Work out the finished part from the listing and answer in its coordinate system (mm). Round coordinates to 2 decimals unless told otherwise and drop trailing zeros. Write each loop counter-clockwise with the first axis right and the second up, starting at its lowest first coordinate (ties: lowest second). Pieces come first, ordered by that corner, then holes. Notation, with made-up numbers: (-34.75, 18) -> (-15.75, 18) arc R13 ccw to (-15.75, 40) -> close; hole circle Ø7 at (89, -24.75). An arc over 180 degrees is marked (long way). One line per item, written item: value.
Autodesk Fusion 360 part; units mm, degrees
sketch "スケッチ1" plane through (0, 0, 0) normal (0, 1, 0) x (1, 0, 0)
  line L0 (0, 0) -> (74, 0)
  line L1 (74, 0) -> (74, -44)
  line L2 (74, -44) -> (0, -44)
  line L3 (0, -44) -> (0, 0)
  dimension "d1" = 74
  dimension "d2" = 44
extrude "押し出し1" add sketch "スケッチ1" along normal blind 2
sketch "スケッチ2" plane through (0, 0, 0) normal (0, -1, 0) x (1, 0, 0)
  line L0 (74, 44) -> (0, 44)
  line L1 (0, 44) -> (0, 0)
  line L2 (0, 0) -> (74, 0)
  line L3 (74, 0) -> (74, 44)
  line L4 (72, 37) -> (74, 37)
  line L5 (74, 37) -> (74, 31)
  line L6 (74, 31) -> (72, 31)
  line L7 (72, 31) -> (72, 37)
  line L8 (74, 25) -> (74, 19)
  line L9 (74, 19) -> (72, 19)
  line L10 (72, 19) -> (72, 25)
  line L11 (72, 25) -> (74, 25)
  line L12 (74, 13) -> (74, 7)
  line L13 (74, 7) -> (72, 7)
  line L14 (72, 7) -> (72, 13)
  line L15 (72, 13) -> (74, 13)
  line L16 (2, 25) -> (2, 19)
  line L17 (2, 31) -> (0, 31)
  line L18 (2, 37) -> (2, 31)
  line L19 (0, 25) -> (2, 25)
  line L20 (2, 13) -> (2, 7)
  line L21 (0, 19) -> (0, 25)
  line L22 (0, 13) -> (2, 13)
  line L23 (2, 7) -> (0, 7)
  line L24 (0, 31) -> (0, 37)
  line L25 (0, 37) -> (2, 37)
  line L26 (0, 7) -> (0, 13)
  line L27 (2, 19) -> (0, 19)
  line L28 (74, 44) -> (72, 44)
  line L29 (72, 44) -> (72, 42)
  line L30 (72, 42) -> (74, 42)
  line L31 (74, 42) -> (74, 44)
  line L32 (0, 44) -> (2, 44)
  line L33 (2, 44) -> (2, 42)
  line L34 (2, 42) -> (0, 42)
  line L35 (0, 42) -> (0, 44)
  line L36 (0, 0) -> (2, 0)
  line L37 (2, 0) -> (2, 2)
  line L38 (2, 2) -> (0, 2)
  line L39 (0, 2) -> (0, 0)
  line L40 (74, 0) -> (72, 0)
  line L41 (72, 0) -> (72, 2)
  line L42 (72, 2) -> (74, 2)
  line L43 (74, 2) -> (74, 0)
  dimension "d7" = 0
  dimension "d8" = -12
  dimension "d9" = 2
  dimension "d10" = 7
  dimension "d11" = 6
  dimension "d12" = 6
  dimension "d13" = 7
  dimension "d16" = -72
  dimension "d17" = 0
extrude "押し出し2" cut sketch "スケッチ2" against normal blind 2 contours L0 L3 L28 L29 L30 L31 | L0 L1 L32 L33 L34 L35 | L3 L4 L5 L6 L7 | L3 L8 L9 L10 L11 | L1 L17 L18 L24 L25 | L3 L12 L13 L14 L15 | L1 L16 L19 L21 L27 | L2 L3 L40 L41 L42 L43 | L1 L20 L22 L23 L26 | L1 L2 L36 L37 L38 L39
sketch "スケッチ3" plane through (0, 0, 0) normal (0, -1, 0) x (1, 0, 0)
  line L0 (74, 31) -> (72, 31)
  line L1 (72, 31) -> (72, 37)
  line L2 (72, 37) -> (74, 37)
  line L3 (74, 37) -> (74, 42)
  line L4 (74, 42) -> (72, 42)
  line L5 (72, 42) -> (72, 44)
  line L6 (72, 44) -> (2, 44)
  line L7 (2, 44) -> (2, 42)
  line L8 (2, 42) -> (0, 42)
  line L9 (0, 42) -> (0, 37)
  line L10 (0, 37) -> (2, 37)
  line L11 (2, 37) -> (2, 31)
  line L12 (2, 31) -> (0, 31)
  line L13 (0, 31) -> (0, 25)
  line L14 (0, 25) -> (2, 25)
  line L15 (2, 25) -> (2, 19)
  line L16 (2, 19) -> (0, 19)
  line L17 (0, 19) -> (0, 13)
  line L18 (0, 13) -> (2, 13)
  line L19 (2, 13) -> (2, 7)
  line L20 (2, 7) -> (0, 7)
  line L21 (0, 7) -> (0, 2)
  line L22 (0, 2) -> (2, 2)
  line L23 (2, 2) -> (2, 0)
  line L24 (2, 0) -> (72, 0)
  line L25 (72, 0) -> (72, 2)
  line L26 (72, 2) -> (74, 2)
  line L27 (74, 2) -> (74, 7)
  line L28 (74, 7) -> (72, 7)
  line L29 (72, 7) -> (72, 13)
  line L30 (72, 13) -> (74, 13)
  line L31 (74, 13) -> (74, 19)
  line L32 (74, 19) -> (72, 19)
  line L33 (72, 19) -> (72, 25)
  line L34 (72, 25) -> (74, 25)
  line L35 (74, 25) -> (74, 31)
  line L36 (0, 44) -> (7, 44)
  line L37 (7, 44) -> (7, 42)
  line L38 (7, 42) -> (0, 42)
  line L39 (0, 42) -> (0, 44)
  line L40 (16, 42) -> (24, 42)
  line L41 (24, 42) -> (24, 44)
  line L42 (24, 44) -> (16, 44)
  line L43 (16, 44) -> (16, 42)
  line L44 (41, 42) -> (41, 44)
  line L45 (33, 42) -> (41, 42)
  line L46 (41, 44) -> (33, 44)
  line L47 (33, 44) -> (33, 42)
  line L48 (58, 42) -> (58, 44)
  line L49 (50, 42) -> (58, 42)
  line L50 (58, 44) -> (50, 44)
  line L51 (50, 44) -> (50, 42)
  line L52 (67, 42) -> (74, 42)
  line L53 (74, 42) -> (74, 44)
  line L54 (74, 44) -> (67, 44)
  line L55 (67, 44) -> (67, 42)
  line L56 (7, 0) -> (0, 0)
  line L57 (41, 2) -> (33, 2)
  line L58 (33, 2) -> (33, 0)
  line L59 (50, 2) -> (50, 0)
  line L60 (24, 2) -> (16, 2)
  line L61 (24, 0) -> (24, 2)
  line L62 (16, 0) -> (24, 0)
  line L63 (7, 2) -> (7, 0)
  line L64 (50, 0) -> (58, 0)
  line L65 (67, 2) -> (67, 0)
  line L66 (0, 0) -> (0, 2)
  line L67 (74, 2) -> (67, 2)
  line L68 (41, 0) -> (41, 2)
  line L69 (58, 2) -> (50, 2)
  line L70 (16, 2) -> (16, 0)
  line L71 (33, 0) -> (41, 0)
  line L72 (67, 0) -> (74, 0)
  line L73 (58, 0) -> (58, 2)
  line L74 (0, 2) -> (7, 2)
  line L75 (74, 0) -> (74, 2)
  line L76 (72, 0) -> (72, 2)
  line L77 (74, 0) -> (72, 0)
  line L78 (2, 2) -> (2, 0)
  line L79 (2, 0) -> (0, 0)
  dimension "d20" = 8
  dimension "d21" = 2
  dimension "d22" = 2
  dimension "d23" = 9
  dimension "d26" = 17
  dimension "d27" = 0
  dimension "d28" = 2
  dimension "d29" = 9
extrude "押し出し3" cut sketch "スケッチ3" against normal blind 2 contours L4 L5 L52 L53 L54 | L5 L6 L52 L54 L55 | L6 L48 L49 L50 L51 | L25 L26 L67 L72 L75 L76 L77 | L6 L44 L45 L46 L47 | L24 L25 L65 L67 L72 L76 | L6 L40 L41 L42 L43 | L24 L59 L64 L69 L73 | L6 L7 L36 L37 L38 | L7 L8 L36 L38 L39 | L24 L57 L58 L68 L71 | L24 L60 L61 L62 L70 | L23 L24 L56 L63 L74 L78 | L22 L23 L56 L66 L74 L78 L79
sketch "スケッチ4" plane through (0, 0, 0) normal (0, -1, 0) x (1, 0, 0)
  line L0 (41, 2) -> (41, 0)
  line L1 (41, 0) -> (50, 0)
  line L2 (50, 0) -> (50, 2)
  line L3 (50, 2) -> (58, 2)
  line L4 (58, 2) -> (58, 0)
  line L5 (58, 0) -> (67, 0)
  line L6 (67, 0) -> (67, 2)
  line L7 (67, 2) -> (74, 2)
  line L8 (74, 2) -> (74, 7)
  line L9 (74, 7) -> (72, 7)
  line L10 (72, 7) -> (72, 13)
  line L11 (72, 13) -> (74, 13)
  line L12 (74, 13) -> (74, 19)
  line L13 (74, 19) -> (72, 19)
  line L14 (72, 19) -> (72, 25)
  line L15 (72, 25) -> (74, 25)
  line L16 (74, 25) -> (74, 31)
  line L17 (74, 31) -> (72, 31)
  line L18 (72, 31) -> (72, 37)
  line L19 (72, 37) -> (74, 37)
  line L20 (74, 37) -> (74, 42)
  line L21 (74, 42) -> (67, 42)
  line L22 (67, 42) -> (67, 44)
  line L23 (67, 44) -> (58, 44)
  line L24 (58, 44) -> (58, 42)
  line L25 (58, 42) -> (50, 42)
  line L26 (50, 42) -> (50, 44)
  line L27 (50, 44) -> (41, 44)
  line L28 (41, 44) -> (41, 42)
  line L29 (41, 42) -> (33, 42)
  line L30 (33, 42) -> (33, 44)
  line L31 (33, 44) -> (24, 44)
  line L32 (24, 44) -> (24, 42)
  line L33 (24, 42) -> (16, 42)
  line L34 (16, 42) -> (16, 44)
  line L35 (16, 44) -> (7, 44)
  line L36 (7, 44) -> (7, 42)
  line L37 (7, 42) -> (0, 42)
  line L38 (0, 42) -> (0, 37)
  line L39 (0, 37) -> (2, 37)
  line L40 (2, 37) -> (2, 31)
  line L41 (2, 31) -> (0, 31)
  line L42 (0, 31) -> (0, 25)
  line L43 (0, 25) -> (2, 25)
  line L44 (2, 25) -> (2, 19)
  line L45 (2, 19) -> (0, 19)
  line L46 (0, 19) -> (0, 13)
  line L47 (0, 13) -> (2, 13)
  line L48 (2, 13) -> (2, 7)
  line L49 (2, 7) -> (0, 7)
  line L50 (0, 7) -> (0, 2)
  line L51 (0, 2) -> (7, 2)
  line L52 (7, 2) -> (7, 0)
  line L53 (7, 0) -> (16, 0)
  line L54 (16, 0) -> (16, 2)
  line L55 (16, 2) -> (24, 2)
  line L56 (24, 2) -> (24, 0)
  line L57 (24, 0) -> (33, 0)
  line L58 (33, 0) -> (33, 2)
  line L59 (33, 2) -> (41, 2)
  line L60 (7, 45) -> (16, 45)
  line L61 (16, 45) -> (16, 44)
  line L62 (16, 44) -> (7, 44)
  line L63 (7, 44) -> (7, 45)
  line L64 (24, 45) -> (33, 45)
  line L65 (33, 45) -> (33, 44)
  line L66 (33, 44) -> (24, 44)
  line L67 (24, 44) -> (24, 45)
  line L68 (41, 45) -> (50, 45)
  line L69 (50, 45) -> (50, 44)
  line L70 (50, 44) -> (41, 44)
  line L71 (41, 44) -> (41, 45)
  line L72 (58, 45) -> (67, 45)
  line L73 (67, 45) -> (67, 44)
  line L74 (67, 44) -> (58, 44)
  line L75 (58, 44) -> (58, 45)
  line L76 (74, 42) -> (75, 42)
  line L77 (75, 42) -> (75, 37)
  line L78 (75, 37) -> (74, 37)
  line L79 (74, 37) -> (74, 42)
  line L80 (74, 31) -> (75, 31)
  line L81 (75, 31) -> (75, 25)
  line L82 (75, 25) -> (74, 25)
  line L83 (74, 25) -> (74, 31)
  line L84 (74, 19) -> (75, 19)
  line L85 (75, 19) -> (75, 13)
  line L86 (75, 13) -> (74, 13)
  line L87 (74, 13) -> (74, 19)
  line L88 (74, 7) -> (75, 7)
  line L89 (75, 7) -> (75, 2)
  line L90 (75, 2) -> (74, 2)
  line L91 (74, 2) -> (74, 7)
  line L92 (58, -1) -> (67, -1)
  line L93 (67, -1) -> (67, 0)
  line L94 (67, 0) -> (58, 0)
  line L95 (58, 0) -> (58, -1)
  line L96 (41, -1) -> (50, -1)
  line L97 (50, -1) -> (50, 0)
  line L98 (50, 0) -> (41, 0)
  line L99 (41, 0) -> (41, -1)
  line L100 (24, 0) -> (33, 0)
  line L101 (33, 0) -> (33, -1)
  line L102 (33, -1) -> (24, -1)
  line L103 (24, -1) -> (24, 0)
  line L104 (16, -1) -> (7, -1)
  line L105 (7, -1) -> (7, 0)
  line L106 (7, 0) -> (16, 0)
  line L107 (16, 0) -> (16, -1)
  line L108 (0, 2) -> (-1, 2)
  line L109 (-1, 2) -> (-1, 7)
  line L110 (-1, 7) -> (0, 7)
  line L111 (0, 7) -> (0, 2)
  line L112 (0, 13) -> (-1, 13)
  line L113 (-1, 13) -> (-1, 19)
  line L114 (-1, 19) -> (0, 19)
  line L115 (0, 19) -> (0, 13)
  line L116 (0, 25) -> (-1, 25)
  line L117 (-1, 25) -> (-1, 31)
  line L118 (-1, 31) -> (0, 31)
  line L119 (0, 31) -> (0, 25)
  line L120 (0, 37) -> (-1, 37)
  line L121 (-1, 37) -> (-1, 42)
  line L122 (-1, 42) -> (0, 42)
  line L123 (0, 42) -> (0, 37)
extrude "押し出し4" add sketch "スケッチ4" against normal blind 2 contours L1 L96 L97 L98 L99 | L57 L100 L101 L102 L103 | L5 L92 L93 L94 L95 | L53 L104 L105 L106 L107 | L8 L88 L89 L90 L91 | L50 L108 L109 L110 L111 | L12 L84 L85 L86 L87 | L46 L112 L113 L114 L115 | L16 L80 L81 L82 L83 | L42 L116 L117 L118 L119 | L20 L76 L77 L78 L79 | L38 L120 L121 L122 L123 | L23 L72 L73 L74 L75 | L35 L60 L61 L62 L63 | L27 L68 L69 L70 L71 | L31 L64 L65 L66 L67
sketch "スケッチ5" plane through (0, 0, 0) normal (0, -1, 0) x (1, 0, 0)
  line L0 (41, 2) -> (41, -1)
  line L1 (41, -1) -> (50, -1)
  line L2 (50, -1) -> (50, 2)
  line L3 (50, 2) -> (58, 2)
  line L4 (58, 2) -> (58, -1)
  line L5 (58, -1) -> (67, -1)
  line L6 (67, -1) -> (67, 2)
  line L7 (67, 2) -> (75, 2)
  line L8 (75, 2) -> (75, 7)
  line L9 (75, 7) -> (72, 7)
  line L10 (72, 7) -> (72, 13)
  line L11 (72, 13) -> (75, 13)
  line L12 (75, 13) -> (75, 19)
  line L13 (75, 19) -> (72, 19)
  line L14 (72, 19) -> (72, 25)
  line L15 (72, 25) -> (75, 25)
  line L16 (75, 25) -> (75, 31)
  line L17 (75, 31) -> (72, 31)
  line L18 (72, 31) -> (72, 37)
  line L19 (72, 37) -> (75, 37)
  line L20 (75, 37) -> (75, 42)
  line L21 (75, 42) -> (67, 42)
  line L22 (67, 42) -> (67, 45)
  line L23 (67, 45) -> (58, 45)
  line L24 (58, 45) -> (58, 42)
  line L25 (58, 42) -> (50, 42)
  line L26 (50, 42) -> (50, 45)
  line L27 (50, 45) -> (41, 45)
  line L28 (41, 45) -> (41, 42)
  line L29 (41, 42) -> (33, 42)
  line L30 (33, 42) -> (33, 45)
  line L31 (33, 45) -> (24, 45)
  line L32 (24, 45) -> (24, 42)
  line L33 (24, 42) -> (16, 42)
  line L34 (16, 42) -> (16, 45)
  line L35 (16, 45) -> (7, 45)
  line L36 (7, 45) -> (7, 42)
  line L37 (7, 42) -> (-1, 42)
  line L38 (-1, 42) -> (-1, 37)
  line L39 (-1, 37) -> (2, 37)
  line L40 (2, 37) -> (2, 31)
  line L41 (2, 31) -> (-1, 31)
  line L42 (-1, 31) -> (-1, 25)
  line L43 (-1, 25) -> (2, 25)
  line L44 (2, 25) -> (2, 19)
  line L45 (2, 19) -> (-1, 19)
  line L46 (-1, 19) -> (-1, 13)
  line L47 (-1, 13) -> (2, 13)
  line L48 (2, 13) -> (2, 7)
  line L49 (2, 7) -> (-1, 7)
  line L50 (-1, 7) -> (-1, 2)
  line L51 (-1, 2) -> (7, 2)
  line L52 (7, 2) -> (7, -1)
  line L53 (7, -1) -> (16, -1)
  line L54 (16, -1) -> (16, 2)
  line L55 (16, 2) -> (24, 2)
  line L56 (24, 2) -> (24, -1)
  line L57 (24, -1) -> (33, -1)
  line L58 (33, -1) -> (33, 2)
  line L59 (33, 2) -> (41, 2)
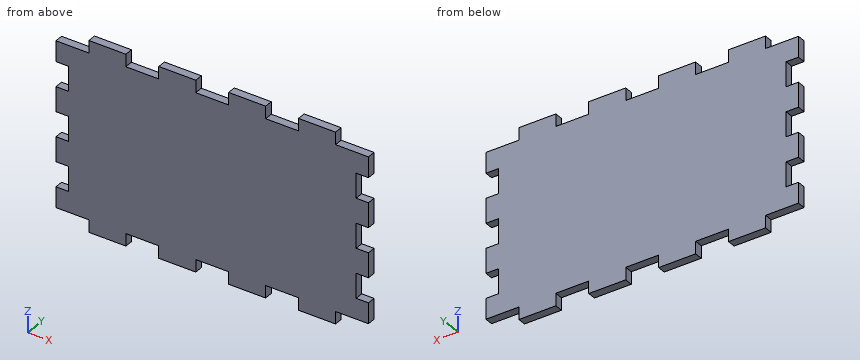
(1) Find section A-A on x = 39.5. Give the vertices of the cut face in (y, z).
Reported:
outline: (0, 2) -> (2, 2) -> (2, 42) -> (0, 42) -> close
(2) Consider probe 1 along Z at (x, y) = (55, 1.45); probe 2 along X at (y, z) = (1.45, 32). Determine where each line is inside the solid, lowest interval first.
Reported:
probe 1: z = 2 to 42
probe 2: x = 2 to 72
(3) Flat-ended cylindrical pins translate along their axes: pin 1 Ø0.6 at (x, y) = (72.5, 0.5) entering from +Z; pin 2 Ø0.6 at (y, z) = (1, 35.5) entering from -X; pin 3 Ø0.6 at (x, y) = (20, 0.5) entering from -Z. Find the tip coordinate at first contact, or state that the pin passes through.
Reported:
pin 1: stops at z = 42
pin 2: stops at x = 2
pin 3: stops at z = 2
(4) Find section B-B on z = 8.5. Give the vertices of the cut face in (x, y).
Reported:
outline: (2, 0) -> (72, 0) -> (72, 2) -> (2, 2) -> close
